Work out the finished part from the listing and answer in its coordinate system (mm). A direction names the side the tool comes from. Round coordinates to 2 decimals unless told otherwise and drop trailing zeros. Order: outer loops, then holes, each group sorted by start corner. A loop starts at its lowest first (then second) coordinate and runs counter-clockwise, first axis right, second up. Notation, with made-up numbers: (78, 79.5) -> (87, 79.5) arc R27 ccw to (87, 98.5) -> close; hole circle Ø5 at (10.25, 13.5). An arc over 180 degrees is marked (long way). Use a Markdown table: item, result. Add a question column.
Item 1: A cutting plane is placed at D-D, the plane z = 9.5. Determine the outline of the cut face in (x, y), plus the area to 3 significant figures.
Item 2: A cutting plane is placed at B-B, the plane x = -2. Determine the outline of the cut face in (y, z), plus the area to 3 significant figures.
Item 3: A cutting plane is placed at C-C, the plane y = 3.75. Determine the outline of the cut face in (x, z).
Item 4: Find the intervals of material crossed by L1, parallel to Z at x = 7, y = 9.25; L2, parallel to Z at x = -27, y = 5.25; L3, parallel to Y at x = -2, z = 19, in increasing order. Write a range as [from, to].
Item 5: A cutting plane is placed at A-A, the plane y = -4. Determine the outline of the cut face in (x, z), plus the area to 3 significant figures.
Item 6: Flat-ended cylindrical pins translate along their axes: P1, Ø8, axis at x = 6.5, z = 23.5, coming from the -Y side; P2, Ø8, axis at x = 2, z = 8.5, coming from the +Y side; P3, Ø17, axis at x = 0.5, z = 16.5, coming from the +Y side. Find the tip coordinate at first contact, or state that the pin passes through.
Item 7: A tool of negligible diameter and unlimited length cuts with its end or side. For faces 1 (the flat face through (-21, 2, 1)), 2 (the flat face through (0, 9, 38.5)), 3 (the flat face through (10.5, 1, 25)), 4 (the flat face through (0, -5, 3)), 5 (the flat face through (-10.5, 1, 25)), from which of +Z, -Z, +X, -X, +Y, -Y can it reach the whole face along a straight path? Write none if from no direction.
Item 8: For a pull along Z with two mould halves and no side action, classify faces 6 (the flat face through (-0.2, 3.2, 4.3)), 7 (the flat face through (12, 2, 4)), 8 (the flat face through (17, 2, 1)) as +Z half, -Z half, draft (parallel to the pull), parting line (faces both ways), or undercut.
from build123d import *

# Parameters (mm, degrees)
SKETCH1_W           = 21
SKETCH1_H           = 4
BOSS_EXTRUDE1_DEPTH = 41.5
SKETCH2_W           = 21
SKETCH2_H           = 3
BOSS_EXTRUDE2_DEPTH = 10
CHAMFER1_SIZE       = 5
BOSS_EXTRUDE3_DEPTH = 21
SKETCH6_W           = 50
SKETCH6_H           = 3
BOSS_EXTRUDE4_DEPTH = 10
CHAMFER3_SIZE       = 2.5
CHAMFER4_SIZE       = 2.5
CHAMFER5_SIZE       = 2.5


with BuildPart() as part:
    # Sketch1 → Boss-Extrude1 (new body)
    with BuildSketch(Plane.XY):
        Rectangle(SKETCH1_W, SKETCH1_H)
    extrude(amount=BOSS_EXTRUDE1_DEPTH)

    # Sketch2 → Boss-Extrude2 (add)
    with BuildSketch(Plane(origin=(0, 2, 0), x_dir=(1, 0, 0), z_dir=(0, 1, 0))):
        with Locations((0, -40)):
            Rectangle(SKETCH2_W, SKETCH2_H)
    extrude(amount=BOSS_EXTRUDE2_DEPTH)

    # Chamfer1
    chamfer1_edges = [part.edges().sort_by_distance(p)[0] for p in [
        (0, 2, 38.5),
    ]]
    chamfer(chamfer1_edges, length=CHAMFER1_SIZE)

    # Sketch4 → Boss-Extrude3 (add)
    with BuildSketch(Plane(origin=(10.5, 0, 0), x_dir=(0, 0, -1), z_dir=(1, 0, 0))):
        Polygon((-35.5, -2), (-41.5, -8), (-41.5, -2), align=None)
        Polygon((0, -2), (0, -8), (-6, -2), align=None)
    extrude(amount=-BOSS_EXTRUDE3_DEPTH)

    # Sketch6 → Boss-Extrude4 (add)
    with BuildSketch(Plane(origin=(0, 2, 0), x_dir=(1, 0, 0), z_dir=(0, 1, 0))):
        with Locations((-4.5, -1.5)):
            Rectangle(SKETCH6_W, SKETCH6_H)
    extrude(amount=BOSS_EXTRUDE4_DEPTH)

    # Chamfer3
    chamfer3_edges = [part.edges().sort_by_distance(p)[0] for p in [
        (0, 2, 3),
    ]]
    chamfer(chamfer3_edges, length=CHAMFER3_SIZE)

    # Chamfer4
    chamfer4_edges = [part.edges().sort_by_distance(p)[0] for p in [
        (-10.5, 2, 1.5),
        (-10.5, 3.25, 3),
    ]]
    chamfer(chamfer4_edges, length=CHAMFER4_SIZE)

    # Chamfer5
    chamfer5_edges = [part.edges().sort_by_distance(p)[0] for p in [
        (10.5, 2, 1.5),
        (10.5, 3.25, 3),
    ]]
    chamfer(chamfer5_edges, length=CHAMFER5_SIZE)


solid = part.part
Reported:
| question | item | result |
|---|---|---|
| 1 | outline | (-10.5, -2) -> (10.5, -2) -> (10.5, 2) -> (-10.5, 2) -> close |
| 1 | area | 84.0 mm² |
| 2 | outline | (-8, 0) -> (12, 0) -> (12, 3) -> (4.5, 3) -> (2, 5.5) -> (2, 33.5) -> (7, 38.5) -> (12, 38.5) -> (12, 41.5) -> (-8, 41.5) -> (-2, 35.5) -> (-2, 6) -> close |
| 2 | area | 278 mm² |
| 3 | outline | (-29.5, 0) -> (20.5, 0) -> (20.5, 3) -> (13, 3) -> (12.25, 3.75) -> (-12.25, 3.75) -> (-13, 3) -> (-29.5, 3) -> close; (-10.5, 35.25) -> (10.5, 35.25) -> (10.5, 41.5) -> (-10.5, 41.5) -> close |
| 4 | L1 | [0, 3], [38.5, 41.5] |
| 4 | L2 | [0, 3] |
| 4 | L3 | [-2, 2] |
| 5 | outline | (-10.5, 0) -> (10.5, 0) -> (10.5, 4) -> (-10.5, 4) -> close; (-10.5, 37.5) -> (10.5, 37.5) -> (10.5, 41.5) -> (-10.5, 41.5) -> close |
| 5 | area | 168 mm² |
| 6 | P1 | y = -2 |
| 6 | P2 | y = 3 |
| 6 | P3 | y = 2 |
| 7 | face 1 | +Z, -Z, -X, -Y |
| 7 | face 2 | +X, -X, +Y |
| 7 | face 3 | +Z, +X, -Y |
| 7 | face 4 | +X, -X, -Y |
| 7 | face 5 | +Z, -X, -Y |
| 8 | face 6 | undercut |
| 8 | face 7 | +Z half |
| 8 | face 8 | draft |
